from build123d import *

# Parameters (mm, degrees)
F2_SIZE  = 0.5
F3_R     = 0.5
F4_R     = 5
F5_DEPTH = 15


with BuildPart() as f1:
    # F0 (on Front) → F1 (revolve)
    with BuildSketch(Plane.XZ):
        with BuildLine():
            Line((0, 32.35), (0, 0))
            Line((0, 0), (173, 0))
            Line((173, 0), (173, 12.5))
            Line((173, 12.5), (170, 12.5))
            Line((170, 12.5), (170, 51))
            Line((170, 51), (155, 51))
            Line((155, 51), (155, 31))
            ThreePointArc((155, 31), (153.242641, 26.757359), (149, 25))
            Line((149, 25), (121, 25))
            ThreePointArc((121, 25), (116.757359, 26.757359), (115, 31))
            Line((115, 31), (115, 38.25))
            Line((115, 38.25), (72.829016, 38.25))
            Line((72.829016, 38.25), (70, 33.35))
            Line((70, 33.35), (70, 32.35))
            Line((70, 32.35), (0, 32.35))
        make_face()
    revolve(axis=Axis((86.5, 0, 0), (1, 0, 0)))

    # F2
    f2_edges = [f1.edges().sort_by_distance(p)[0] for p in [
        (0, 0, -32.35),
        (115, 0, -38.25),
        (155, 0, -51),
        (170, 0, -51),
    ]]
    chamfer(f2_edges, length=F2_SIZE)

    # F3
    f3_edges = [f1.edges().sort_by_distance(p)[0] for p in [
        (70, 0, -32.35),
        (170, 0, -12.5),
    ]]
    fillet(f3_edges, radius=F3_R)

    # F4 (on face) → F5 (cut, through all)
    with BuildSketch(Plane.YZ.offset(170)):
        with Locations((0, 38.25)):
            Circle(F4_R)
        with Locations((-27.046834, 27.046834)):
            Circle(F4_R)
        with Locations((-38.25, 0)):
            Circle(F4_R)
        with Locations((-27.046834, -27.046834)):
            Circle(F4_R)
        with Locations((0, -38.25)):
            Circle(F4_R)
        with Locations((27.046834, -27.046834)):
            Circle(F4_R)
        with Locations((38.25, 0)):
            Circle(F4_R)
        with Locations((27.046834, 27.046834)):
            Circle(F4_R)
    extrude(amount=-F5_DEPTH, mode=Mode.SUBTRACT)


solid = f1.part
Can you work these out from the model? Positions are in its coordinate system, mm. A direction names the side the tool comes from. Coordinates: 2 decimals unless noted, no trailing zeros. Loops run counter-clockwise (first coordinate to the right, second up) from the corner with the lowest first, then second, coordinate; pieces in that order, holes last. Notation, with made-up numbers: M 12,-24.75 L 30,-24.75 A31 ccw 30,8.25 Z; hole C -20.5,50.5 d5. An arc over 180 degrees is marked long. Answer as CSV lines item,"result". Start each with the question number.
1. Suppose I cut it at A-A, the plane y = 0. Count the separate pieces of the cut face and the enclosed holes in it, plus the area to 3 significant figures.
2. For faces 1 (the face through (93.373, 23.275, -30.354)), 2 (the face through (162.402, 49.787, -11.056)), 3 (the face through (162.605, -43.245, 0.22)), 4 (the face through (0, 0, 0)), 5 (the face through (115, -31, 6)), which set-ups out of +Z, -Z, +X, -X, +Y, -Y let a thin tool reach every point of the face, with its end or its side?
3. Suppose I cut it at C-C, the plane x = 32. List the corners of the cut face in (y, z) for me, plus the area to 3 significant figures.
4. For pin 1 Ø6 at (y, z) = (38.25, 0) entering from -X; pin 2 Ø16 at (y, z) = (-27.05, -27.05) entering from +X; pin 3 Ø8 at (y, z) = (0, 38.25) entering from +X, each with a flat end and sliding along its axis, tell me the tip position at first contact or that it passes through.
5. If I drill on probe 1 along Z at (x, y) = (66, -20.5); probe 2 along X at (y, z) = (-36, 33); probe 3 along X at (y, z) = (-16.5, 27), over which ranges is the centre line in solid material (lowest first)? Write a range as [from, to].
6. Thinking about a two-plate mould opening in X: for faces 6 (the face through (162.6, -0.7, 43.2)), 7 (the face through (70, 22.08, 24.55)), 8 (the face through (134.804, -7.509, 23.846)), which applies, +X half, -X half, draft (parallel to the pull), parting line (faces both ways), or undercut?
7. Suppose I cut it at B-B, the plane x = 92. List the corners of the cut face in (y, z) for me.
Output:
1,separate pieces,"3"
1,enclosed holes,"0"
1,area,"11,300 mm^2"
2,face 1,"-X"
2,face 2,"+X, -X"
2,face 3,"+X"
2,face 4,"+Z, -Z, -X, +Y, -Y"
2,face 5,"none"
3,outline,"C 0,0 d64.7"
3,area,"3,290 mm^2"
4,pin 1,"stops at x = 71.1"
4,pin 2,"stops at x = 170"
4,pin 3,"stops at x = 115"
5,probe 1,"z = [-25.03, 25.03]"
5,probe 2,"x = [155, 170]"
5,probe 3,"x = [0, 115], [155, 170]"
6,face 6,"draft"
6,face 7,"-X half"
6,face 8,"undercut"
7,outline,"C 0,0 d76.5"
